Input: part model. Units: mm. Frame: model coordinates. Face numbers are marked on the shaded views. A direction names the side the tool comes from. Coordinates: 2 decimals unless noted, no trailing zeros. Write each loop counter-clockwise with the first axis right and the second up, starting at its lowest first coordinate (ties: lowest second). Pieces come first, ordered by that corner, then holes.
1) Pin query (flat end, axial travel): pin 1 Ø0.5 at (y, z) = (1.5, 1) entering from -X; pin 2 Ø0.8 at (y, z) = (0, 1) entering from +X. Return the tip coordinate at first contact, or that it passes through.
2) Section query A-A (z = 1.1). Output: boundary loops of the cut face in (x, y), then the cut area to 3 significant figures.
3) Section query D-D (x = 2.5). Output: boundary loops of the cut face in (y, z), then the cut area to 3 significant figures.
4) Section query B-B (y = -2). Output: boundary loops of the cut face in (x, z).
5) Section query C-C (z = 1.65). Output: boundary loops of the cut face in (x, y).
6) Set-up query: the marked faces 1, 2 and 3. Return all of +Z, -Z, +X, -X, +Y, -Y with unobstructed straight access to the full face (end or side cutting, diameter ignored); none if empty.
7) Line query: L1, parallel to X at y = 0.7, z = 0.35; L2, parallel to X at y = -0.95, z = 0.15; L3, parallel to Z at x = -3.5, y = -0.5. Output: solid intervals per line, ascending.
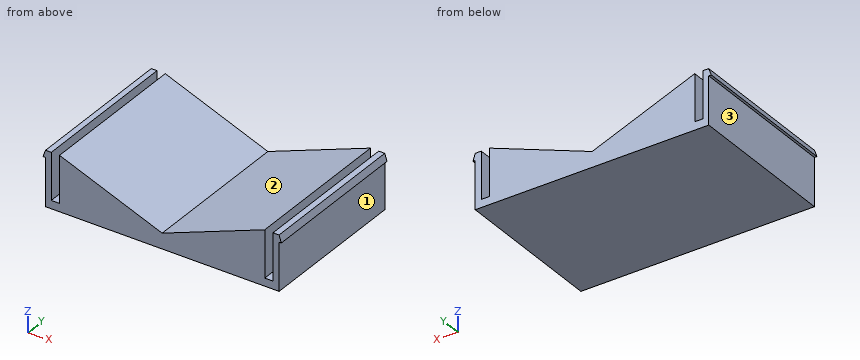
from build123d import *

# Parameters (mm, degrees)
F0_W     = 6.64972
F0_H     = 4.99872
F1_DEPTH = 1.778
F3_DEPTH = 25.4
F4_W     = 0.26797
F4_H     = 1.5150946512
F4_H_2   = 0.2629053488
F4_H_3   = 0.255633
F4_H_4   = 1.522367
F5_DEPTH = 4.99872
F6_W     = 0.0717422777
F6_H     = 1.5494
F6_W_2   = 0.0822888074
F7_DEPTH = 25.4


with BuildPart() as f1:
    # F0 (on Top) → F1 (new body)
    with BuildSketch(Plane.XY):
        with Locations((0, 0.1761515194)):
            Rectangle(F0_W, F0_H)
    extrude(amount=F1_DEPTH)

    # F2 (on face) → F3 (cut)
    with BuildSketch(Plane.XZ.offset(2.3232084806)):
        Polygon((-3.32486, 1.778), (0, 0.4989000154), (3.32486, 1.778), align=None)
    extrude(amount=-F3_DEPTH, mode=Mode.SUBTRACT)

    # F4 (on face) → F5 (join, through all)
    with BuildSketch(Plane.XZ.offset(2.3232084806)):
        with Locations((-3.726815, 1.0204526744)):
            Rectangle(F4_W, F4_H)
        with Locations((-3.726815, 0.1314526744)):
            Rectangle(F4_W, F4_H_2)
        with Locations((-3.458845, 0.1314526744)):
            Rectangle(F4_W, F4_H_2)
        with Locations((3.458845, 0.1278165)):
            Rectangle(F4_W, F4_H_3)
        with Locations((3.726815, 0.1278165)):
            Rectangle(F4_W, F4_H_3)
        with Locations((3.726815, 1.0168165)):
            Rectangle(F4_W, F4_H_4)
    extrude(amount=-F5_DEPTH)

    # F6 (on face) → F7 (cut)
    with BuildSketch(Plane(origin=(0, 2.6755115194, 0), x_dir=(-1, 0, 0), z_dir=(0, 1, 0))):
        with Locations((-3.8249288612, 0.7747)):
            Rectangle(F6_W, F6_H)
        Polygon((-3.8608, 1.778), (-3.8608, 1.5494), (-3.7890577223, 1.778), align=None)
        Polygon((3.7785111926, 1.778), (3.8608, 1.5494), (3.8608, 1.778), align=None)
        with Locations((3.8196555963, 0.7747)):
            Rectangle(F6_W_2, F6_H)
    extrude(amount=-F7_DEPTH, mode=Mode.SUBTRACT)


solid = f1.part
Answer:
1. pin 1: stops at x = -3.78
1. pin 2: stops at x = 3.79
2. outline: (-3.78, -2.32) - (-3.59, -2.32) - (-3.59, 2.68) - (-3.78, 2.68) - close; (-3.32, -2.32) - (-1.56, -2.32) - (-1.56, 2.68) - (-3.32, 2.68) - close; (1.56, -2.32) - (3.32, -2.32) - (3.32, 2.68) - (1.56, 2.68) - close; (3.59, -2.32) - (3.79, -2.32) - (3.79, 2.68) - (3.59, 2.68) - close
2. area: 19.5 mm2
3. outline: (-2.32, 0) - (2.68, 0) - (2.68, 1.46) - (-2.32, 1.46) - close
3. area: 7.30 mm2
4. outline: (-3.86, 1.55) - (-3.78, 1.55) - (-3.78, 0) - (3.79, 0) - (3.79, 1.55) - (3.86, 1.55) - (3.79, 1.78) - (3.59, 1.78) - (3.59, 0.26) - (3.32, 0.26) - (3.32, 1.78) - (0, 0.5) - (-3.32, 1.78) - (-3.32, 0.26) - (-3.59, 0.26) - (-3.59, 1.78) - (-3.78, 1.78) - close
5. outline: (-3.82, -2.32) - (-3.59, -2.32) - (-3.59, 2.68) - (-3.82, 2.68) - close; (-3.32, -2.32) - (-2.99, -2.32) - (-2.99, 2.68) - (-3.32, 2.68) - close; (2.99, -2.32) - (3.32, -2.32) - (3.32, 2.68) - (2.99, 2.68) - close; (3.59, -2.32) - (3.83, -2.32) - (3.83, 2.68) - (3.59, 2.68) - close
6. face 1: -Z, +X, +Y, -Y
6. face 2: +Z, +Y, -Y
6. face 3: -Z, -X, +Y, -Y
7. L1: x = -3.78 to -3.59, -3.32 to 3.32, 3.59 to 3.79
7. L2: x = -3.78 to 3.79
7. L3: z = 0 to 0.26
